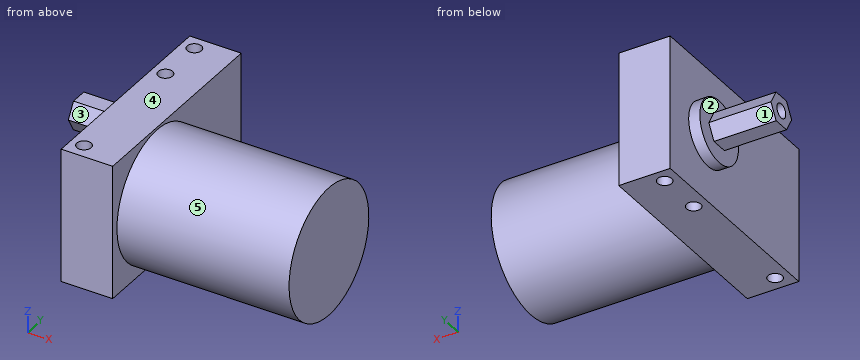
from build123d import *

# Parameters (mm, degrees)
SKETCH_1_W          = 30
SKETCH_1_H          = 46.6
SKETCH_1_R          = 7
SKETCH_1_R_2        = 1.6
EXTRUDE_1_DEPTH     = 11.5
SKETCH_1_3_R        = 7
EXTRUDE_2_DEPTH     = 2.5
SKETCH_1_4_R        = 1.6
EXTRUDE_3_DEPTH     = 16.4
SKETCH_1_5_R        = 1.6
EXTRUDE_4_DEPTH     = 10.4
SKETCH_2_R          = 14.45
EXTRUDE_5_DEPTH     = 38.5
SKETCH_3_R          = 1.6
CUT_EXTRUDE_1_DEPTH = 6
SKETCH_4_R          = 1.6
CUT_EXTRUDE_2_DEPTH = 3


with BuildPart() as part:
    # Sketch 1 → Extrude 1 (new body)
    # profile 1 of 4: a face of its own
    with BuildSketch(Plane(origin=(0, 0, 0), x_dir=(0, 0, -1), z_dir=(1, 0, 0))):
        with Locations((15, 23.3)):
            Rectangle(SKETCH_1_W, SKETCH_1_H)
        with Locations((15, 32.9)):
            Circle(SKETCH_1_R, mode=Mode.SUBTRACT)
    # profile 2 of 4: a face of its own
    with BuildSketch(Plane(origin=(0, 0, 0), x_dir=(0, 0, -1), z_dir=(1, 0, 0))):
        with Locations((15, 32.9)):
            Circle(SKETCH_1_R)
        Polygon((18.25, 31.023611625), (18.25, 34.776388375), (15, 36.65277675), (11.75, 34.776388375), (11.75, 31.023611625), (15, 29.14722325), align=None, mode=Mode.SUBTRACT)
    # profile 3 of 4: a face of its own
    with BuildSketch(Plane(origin=(0, 0, 0), x_dir=(0, 0, -1), z_dir=(1, 0, 0))):
        Polygon((15, 29.14722325), (18.25, 31.023611625), (18.25, 34.776388375), (15, 36.65277675), (11.75, 34.776388375), (11.75, 31.023611625), align=None)
        with Locations((15, 32.9)):
            Circle(SKETCH_1_R_2, mode=Mode.SUBTRACT)
    # profile 4 of 4: a face of its own
    with BuildSketch(Plane(origin=(0, 0, 0), x_dir=(0, 0, -1), z_dir=(1, 0, 0))):
        with Locations((15, 32.9)):
            Circle(SKETCH_1_R_2)
    extrude(amount=EXTRUDE_1_DEPTH)

    # Sketch 1_3 → Extrude 2 (add)
    with BuildSketch(Plane(origin=(0, 0, 0), x_dir=(0, 0, -1), z_dir=(1, 0, 0))):
        with Locations((15, 32.9)):
            Circle(SKETCH_1_3_R)
        Polygon((18.25, 31.023611625), (18.25, 34.776388375), (15, 36.65277675), (11.75, 34.776388375), (11.75, 31.023611625), (15, 29.14722325), align=None, mode=Mode.SUBTRACT)
    extrude(amount=-EXTRUDE_2_DEPTH)

    # Sketch 1_4 → Extrude 3 (add)
    with BuildSketch(Plane(origin=(0, 0, 0), x_dir=(0, 0, -1), z_dir=(1, 0, 0))):
        Polygon((15, 29.14722325), (18.25, 31.023611625), (18.25, 34.776388375), (15, 36.65277675), (11.75, 34.776388375), (11.75, 31.023611625), align=None)
        with Locations((15, 32.9)):
            Circle(SKETCH_1_4_R, mode=Mode.SUBTRACT)
    extrude(amount=-EXTRUDE_3_DEPTH)

    # Sketch 1_5 → Extrude 4 (add)
    with BuildSketch(Plane(origin=(0, 0, 0), x_dir=(0, 0, -1), z_dir=(1, 0, 0))):
        with Locations((15, 32.9)):
            Circle(SKETCH_1_5_R)
    extrude(amount=-EXTRUDE_4_DEPTH)

    # Sketch 2 → Extrude 5 (add)
    with BuildSketch(Plane(origin=(11.5, 0, 0), x_dir=(0, 0, -1), z_dir=(1, 0, 0))):
        with Locations((15, 16)):
            Circle(SKETCH_2_R)
    extrude(amount=EXTRUDE_5_DEPTH)

    # Sketch 3 → Cut-Extrude 1 (cut)
    with BuildSketch(Plane.XY):
        with Locations((3, 43.4)):
            Circle(SKETCH_3_R)
        with Locations((3, 32.9)):
            Circle(SKETCH_3_R)
        with Locations((3, 3.4)):
            Circle(SKETCH_3_R)
    extrude(amount=-CUT_EXTRUDE_1_DEPTH, mode=Mode.SUBTRACT)

    # Sketch 4 → Cut-Extrude 2 (cut)
    with BuildSketch(Plane(origin=(0, 0, -30), x_dir=(-1, 0, 0), z_dir=(0, 0, -1))):
        with Locations((-3.2, 43.4)):
            Circle(SKETCH_4_R)
        with Locations((-3.2, 32.9)):
            Circle(SKETCH_4_R)
        with Locations((-3.2, 3.4)):
            Circle(SKETCH_4_R)
    extrude(amount=-CUT_EXTRUDE_2_DEPTH, mode=Mode.SUBTRACT)


solid = part.part
Can you work these out from the model? Positions are in its coordinate system, mm. Face numbers are marked on the shaded views. A direction names the side the tool comes from. Give positions to 0.01 mm unless a question says otherwise; leave off trailing zeros. Order: outer loops, then holes, each group sorted by start corner. A loop starts at its lowest first (then second) coordinate and runs counter-clockwise, first axis right, second up. Notation, with made-up numbers: M 33,5 L 85,5 A22 ccw 85,13 Z; hole C -17,-14.5 d5. An arc over 180 degrees is marked long. Use a Markdown table: item, result. Add a question column.
Item 1: Suppose I cut it at C-C (z = -2.5). List the corners of the cut face in (x, y) for me, then the cut area to 3 significant figures.
Item 2: Will these pins go through, and if not, where does the flat tip stop? pin 1 (6 mm diameter, centred on x = 23.5, y = 5.5, fed in from +Z); pin 2 (6 mm diameter, centred on x = -2, y = 5, fed in from -Z); pin 3 (1.9 mm diameter, centred on y = 32.9, z = -15, fed in from +X); pin 4 (4 mm diameter, centred on x = 42.5, y = 30, fed in from -Z).
Item 3: For the marked faces 1, 2, 3, 4 and 5, which set-ups out of +Z, -Z, +X, -X, +Y, -Y let a thin tool reach every point of the face, with its end or its side?
Item 4: Suppose I cut it at B-B (z = -19.5). List the corners of the cut face in (x, y) for me, then the cut area to 3 significant figures.
Item 5: Suppose I cut it at D-D (x = 3.2). List the corners of the cut face in (y, z) for me, then the cut area to 3 significant figures.
Item 6: Suppose I cut it at A-A (y = 43.4). List the corners of the cut face in (x, z) for me.
Item 7: If I drill on L1, parallel to Y at x = 3.2, z = -28.8; L2, parallel to X at y = 7, z = -21.5; L3, parallel to X at y = 29.5, z = -23, over which ranges is the centre line in solid material (lowest first)? Write a range as [from, to].
Answer sheet:
| question | item | result |
|---|---|---|
| 1 | outline | M 0,0 L 11.5,0 L 11.5,8.75 L 50,8.75 L 50,23.25 L 11.5,23.25 L 11.5,46.6 L 0,46.6 Z; hole C 3,3.4 d3.2; hole C 3,32.9 d3.2; hole C 3,43.4 d3.2 |
| 1 | area | 1,070 mm² |
| 2 | pin 1 | stops at z = -2.65 |
| 2 | pin 2 | stops at z = -30 |
| 2 | pin 3 | stops at x = 11.5 |
| 2 | pin 4 | stops at z = -23.05 |
| 3 | face 1 | -Z, -X, +Y |
| 3 | face 2 | -X |
| 3 | face 3 | +Z, -X, -Y |
| 3 | face 4 | +Z, +X, -X, +Y, -Y |
| 3 | face 5 | +X |
| 4 | outline | M -2.5,27.54 L 0,27.54 L 0,0 L 11.5,0 L 11.5,2.27 L 50,2.27 L 50,29.73 L 11.5,29.73 L 11.5,46.6 L 0,46.6 L 0,38.26 L -2.5,38.26 Z |
| 4 | area | 1,620 mm² |
| 5 | outline | M 0,-30 L 1.8,-30 L 1.8,-27 L 5,-27 L 5,-30 L 31.3,-30 L 31.3,-27 L 34.5,-27 L 34.5,-30 L 41.8,-30 L 41.8,-27 L 45,-27 L 45,-30 L 46.6,-30 L 46.6,0 L 44.99,0 L 44.99,-6 L 41.81,-6 L 41.81,0 L 34.49,0 L 34.49,-6 L 31.31,-6 L 31.31,0 L 4.99,0 L 4.99,-6 L 1.81,-6 L 1.81,0 L 0,0 Z |
| 5 | area | 1,310 mm² |
| 6 | outline | M 0,-30 L 1.6,-30 L 1.6,-27 L 4.8,-27 L 4.8,-30 L 11.5,-30 L 11.5,0 L 4.6,0 L 4.6,-6 L 1.4,-6 L 1.4,0 L 0,0 Z |
| 7 | L1 | y = [0, 1.8], [5, 31.3], [34.5, 41.8], [45, 46.6] |
| 7 | L2 | x = [0, 50] |
| 7 | L3 | x = [0, 11.5] |
